Geometry check sheet. Reference: the model listing, model coordinates, mm. A direction names the side the tool comes from. Coordinates: 2 decimals unless noted, no trailing zeros. Loops run counter-clockwise (first coordinate to the right, second up) from the corner with the lowest first, then second, coordinate; pieces in that order, holes last.
from build123d import *

# Parameters (mm, degrees)
SKETCH1_W           = 41.1
SKETCH1_H           = 17.664696838
BOSS_EXTRUDE1_DEPTH = 12
SKETCH2_W           = 41.1
SKETCH2_H           = 17.664696838
SKETCH2_R           = 4.75
BOSS_EXTRUDE2_DEPTH = 1.5
CHAMFER2_SIZE       = 4
SKETCH3_W           = 33.1
SKETCH3_H           = 13.5
BOSS_EXTRUDE3_DEPTH = 75.2176516
SKETCH4_W           = 33.1
SKETCH4_H           = 20
BOSS_EXTRUDE4_DEPTH = 2.5
CUT_EXTRUDE1_REACH  = 100.057
SKETCH5_R           = 2.25
RIB1_REACH          = 94.253
SKETCH6_WALL_W      = 208.867644448
SKETCH6_WALL_H      = 8
RIB2_REACH          = 94.253
SKETCH7_WALL_W      = 208.867644448
SKETCH7_WALL_H      = 8


with BuildPart() as part:
    # Sketch1 → Boss-Extrude1 (new body)
    with BuildSketch(Plane.XY):
        Rectangle(SKETCH1_W, SKETCH1_H)
        Polygon((-12.7, -7.332348419), (-6.35, -3.666174209), (0, -7.332348419), (6.35, -3.666174209), (12.7, -7.332348419), (19.05, -3.666174209), (19.05, 3.666174209), (12.7, 7.332348419), (6.35, 3.666174209), (0, 7.332348419), (-6.35, 3.666174209), (-12.7, 7.332348419), (-19.05, 3.666174209), (-19.05, -3.666174209), align=None, mode=Mode.SUBTRACT)
    extrude(amount=BOSS_EXTRUDE1_DEPTH)

    # Sketch2 → Boss-Extrude2 (add)
    with BuildSketch(Plane(origin=(0, 0, 0), x_dir=(-1, 0, 0), z_dir=(0, 0, -1))):
        Rectangle(SKETCH2_W, SKETCH2_H)
        Polygon((19.05, -3.666174209), (12.7, -7.332348419), (6.35, -3.666174209), (0, -7.332348419), (-6.35, -3.666174209), (-12.7, -7.332348419), (-19.05, -3.666174209), (-19.05, 3.666174209), (-12.7, 7.332348419), (-6.35, 3.666174209), (0, 7.332348419), (6.35, 3.666174209), (12.7, 7.332348419), (19.05, 3.666174209), align=None, mode=Mode.SUBTRACT)
        Polygon((6.35, -3.666174209), (6.35, 3.666174209), (12.7, 7.332348419), (19.05, 3.666174209), (19.05, -3.666174209), (12.7, -7.332348419), align=None)
        with Locations((12.7, 0)):
            Circle(SKETCH2_R, mode=Mode.SUBTRACT)
        Polygon((6.35, -3.666174209), (6.35, 3.666174209), (0, 7.332348419), (-6.35, 3.666174209), (-6.35, -3.666174209), (0, -7.332348419), align=None)
        Circle(SKETCH2_R, mode=Mode.SUBTRACT)
        Polygon((-6.35, 3.666174209), (-6.35, -3.666174209), (-12.7, -7.332348419), (-19.05, -3.666174209), (-19.05, 3.666174209), (-12.7, 7.332348419), align=None)
        with Locations((-12.7, 0)):
            Circle(SKETCH2_R, mode=Mode.SUBTRACT)
    extrude(amount=BOSS_EXTRUDE2_DEPTH)

    # Chamfer2
    chamfer2_edges = [part.edges().sort_by_distance(p)[0] for p in [
        (-20.55, -8.832348419, 5.25),
        (-20.55, 8.832348419, 5.25),
        (20.55, 8.832348419, 5.25),
        (20.55, -8.832348419, 5.25),
    ]]
    chamfer(chamfer2_edges, length=CHAMFER2_SIZE)

    # Sketch3 → Boss-Extrude3 (add)
    with BuildSketch(Plane.XZ.offset(8.832348419)):
        with Locations((0, 5.25)):
            Rectangle(SKETCH3_W, SKETCH3_H)
    extrude(amount=BOSS_EXTRUDE3_DEPTH)

    # Sketch4 → Boss-Extrude4 (add)
    with BuildSketch(Plane.XZ.offset(84.050000019)):
        with Locations((0, 22)):
            Rectangle(SKETCH4_W, SKETCH4_H)
        with Locations((0, -11.5)):
            Rectangle(SKETCH4_W, SKETCH4_H)
    extrude(amount=-BOSS_EXTRUDE4_DEPTH)

    # Sketch5 → Cut-Extrude1 (cut, up to next)
    with BuildSketch(Plane(origin=(0, -81.550000019, 0), x_dir=(1, 0, 0), z_dir=(0, 1, 0)), mode=Mode.PRIVATE) as cut_extrude1_sk1:
        with Locations(Location((-10.55, -26, 0), (0, 0, 270))):
            Circle(SKETCH5_R)
    cut_extrude1_tool1 = extrude(cut_extrude1_sk1.sketch, amount=-CUT_EXTRUDE1_REACH, mode=Mode.PRIVATE) & part.part
    # Sketch5 → Cut-Extrude1 (cut, up to next)
    with BuildSketch(Plane(origin=(0, -81.550000019, 0), x_dir=(1, 0, 0), z_dir=(0, 1, 0)), mode=Mode.PRIVATE) as cut_extrude1_sk2:
        with Locations(Location((10.55, -26, 0), (0, 0, 270))):
            Circle(SKETCH5_R)
    cut_extrude1_tool2 = extrude(cut_extrude1_sk2.sketch, amount=-CUT_EXTRUDE1_REACH, mode=Mode.PRIVATE) & part.part
    # Sketch5 → Cut-Extrude1 (cut, up to next)
    with BuildSketch(Plane(origin=(0, -81.550000019, 0), x_dir=(1, 0, 0), z_dir=(0, 1, 0)), mode=Mode.PRIVATE) as cut_extrude1_sk3:
        with Locations(Location((10.55, 15.5, 0), (0, 0, 270))):
            Circle(SKETCH5_R)
    cut_extrude1_tool3 = extrude(cut_extrude1_sk3.sketch, amount=-CUT_EXTRUDE1_REACH, mode=Mode.PRIVATE) & part.part
    # Sketch5 → Cut-Extrude1 (cut, up to next)
    with BuildSketch(Plane(origin=(0, -81.550000019, 0), x_dir=(1, 0, 0), z_dir=(0, 1, 0)), mode=Mode.PRIVATE) as cut_extrude1_sk4:
        with Locations(Location((-10.55, 15.5, 0), (0, 0, 270))):
            Circle(SKETCH5_R)
    cut_extrude1_tool4 = extrude(cut_extrude1_sk4.sketch, amount=-CUT_EXTRUDE1_REACH, mode=Mode.PRIVATE) & part.part
    add(cut_extrude1_tool1.solids().sort_by_distance((-10.55, -81.55, 26))[0], mode=Mode.SUBTRACT)
    add(cut_extrude1_tool2.solids().sort_by_distance((10.55, -81.55, 26))[0], mode=Mode.SUBTRACT)
    add(cut_extrude1_tool3.solids().sort_by_distance((10.55, -81.55, -15.5))[0], mode=Mode.SUBTRACT)
    add(cut_extrude1_tool4.solids().sort_by_distance((-10.55, -81.55, -15.5))[0], mode=Mode.SUBTRACT)

    # Sketch6 wall → Rib1 (add, up to next)
    with BuildSketch(Plane(origin=(0, -71.550000019, 17), x_dir=(0, 0.894427191, -0.4472135955), z_dir=(0, 0.4472135955, 0.894427191)), mode=Mode.PRIVATE) as rib1_sk1:
        Rectangle(SKETCH6_WALL_W, SKETCH6_WALL_H)
    rib1_tool1 = extrude(rib1_sk1.sketch, amount=-RIB1_REACH, mode=Mode.PRIVATE) - part.part
    add(rib1_tool1.solids().sort_by_distance((0, -71.550000019, 17))[0])

    # Sketch7 wall → Rib2 (add, up to next)
    with BuildSketch(Plane(origin=(0, -71.550000019, -6.5), x_dir=(0, -0.894427191, -0.4472135955), z_dir=(0, 0.4472135955, -0.894427191)), mode=Mode.PRIVATE) as rib2_sk1:
        Rectangle(SKETCH7_WALL_W, SKETCH7_WALL_H)
    rib2_tool1 = extrude(rib2_sk1.sketch, amount=-RIB2_REACH, mode=Mode.PRIVATE) - part.part
    add(rib2_tool1.solids().sort_by_distance((0, -71.550000019, -6.5))[0])


solid = part.part
1) Section check C-C on x = -3. Record the cut outline in (y, z), and give its area (3 significant figures).
Data:
outline: (-84.05, -21.5) - (-81.55, -21.5) - (-81.55, -11.5) - (-61.55, -1.5) - (-3.68, -1.5) - (-3.68, 0) - (-5.6, 0) - (-5.6, 12) - (-61.55, 12) - (-81.55, 22) - (-81.55, 32) - (-84.05, 32) - close; (3.68, -1.5) - (8.83, -1.5) - (8.83, 12) - (5.6, 12) - (5.6, 0) - (3.68, 0) - close
area: 1,410 mm2
2) Section check B-B on y = 0. Record the cut outline in (x, z).
Data:
outline: (-20.55, -1.5) - (-17.45, -1.5) - (-17.45, 0) - (-19.05, 0) - (-19.05, 12) - (-20.55, 12) - close; (-7.95, -1.5) - (-4.75, -1.5) - (-4.75, 0) - (-7.95, 0) - close; (4.75, -1.5) - (7.95, -1.5) - (7.95, 0) - (4.75, 0) - close; (17.45, -1.5) - (20.55, -1.5) - (20.55, 12) - (19.05, 12) - (19.05, 0) - (17.45, 0) - close
3) Access from +Z, -Z, +X, -X, +Y, -Y to the whole of each face (thin tool, end or side, straight path). Record for faces 1 (the cylindrical face through (-12.546, -82.783, -14.462)), 2 (the flat face through (-4, -75, 16)), 3 (the flat face through (-9.569, -5.525, 5.916)), 4 (the flat face through (0, -81.55, -14)), 5 (the flat face through (18.52, -6.86, 5.34)).
Data:
face 1: +Y, -Y
face 2: +Z, -X, +Y
face 3: +Z
face 4: -Z, +Y
face 5: +Z, -Z, +X, -Y
4) Section check A-A on z = 26. Record the cut outline in (x, y).
Data:
outline: (-16.55, -84.05) - (-12.8, -84.05) - (-12.8, -81.55) - (-16.55, -81.55) - close; (-8.3, -84.05) - (8.3, -84.05) - (8.3, -81.55) - (-8.3, -81.55) - close; (12.8, -84.05) - (16.55, -84.05) - (16.55, -81.55) - (12.8, -81.55) - close
5) Mould release check, pull along X, two halves, no side actions. Record for faces 6 (the cylindrical face through (11.226, -82.783, 28.146)), 7 (the flat face through (-0.06, -71.69, 17.07)), 8 (the flat face through (4, -75, -4)): +X half, -X half, draft (parallel to the pull), parting line (faces both ways), or undercut.
Data:
face 6: undercut
face 7: draft
face 8: +X half
6) Depth check by flat-ended pin: pin 1 (2.5 mm diameter, centred on x = -10.55, z = -15.5, fed in from +Y); pin 2 (12.5 mm diameter, centred on x = 12.7, y = 0, fed in from -Z); pin 3 (6 mm diameter, centred on y = -37.5, z = 10.5, fed in from -X); pin 4 (5 mm diameter, centred on x = 10.55, z = -15.5, fed in from +Y). Enter the tip coordinate at first touch or a pass-through.
Data:
pin 1: passes through
pin 2: stops at z = -1.5
pin 3: stops at x = -16.55
pin 4: stops at y = -81.55
7) Material ranges on probe 1 along X at (y, z) = (-83.4, -15.5); probe 2 along Y at (x, z) = (4.5, 7.5); probe 3 along X at (y, z) = (-82, -15), recorded low to high.
Data:
probe 1: x = -16.55 to -12.8, -8.3 to 8.3, 12.8 to 16.55
probe 2: y = -84.05 to -4.73, 4.73 to 8.83
probe 3: x = -16.55 to -12.74, -8.36 to 8.36, 12.74 to 16.55
8) Section check D-D on z = -5.5. Record the cut outline in (x, y), and give its area (3 significant figures).
Data:
outline: (-16.55, -84.05) - (16.55, -84.05) - (16.55, -81.55) - (4, -81.55) - (4, -69.55) - (-4, -69.55) - (-4, -81.55) - (-16.55, -81.55) - close
area: 179 mm2
